```python
from build123d import *

# Parameters (mm, degrees)
F1_DEPTH = 2.54


with BuildPart() as f1:
    # F0 (on Top) → F1 (new body)
    with BuildSketch(Plane.XY):
        with BuildLine():
            ThreePointArc((-11.5484487595, -6.6675), (-11.5484487595, 6.6675), (0, 13.335))
            Line((0, 13.335), (0, 41.5238420934))
            ThreePointArc((0, 41.5238420934), (-3.4923003016, 43.8671250358), (-2.6478593482, 47.9870832663))
            ThreePointArc((-2.6478593482, 47.9870832663), (-4.0365508418, 49.1893730793), (-4.9196396151, 50.8))
            Line((-4.9196396151, 50.8), (-7.62, 50.8))
            ThreePointArc((-7.62, 50.8), (-13.2627477276, 7.6572509707), (-47.8040905122, -18.8008864232))
            Line((-47.8040905122, -18.8008864232), (-46.456170155, -21.1355529664))
            ThreePointArc((-46.456170155, -21.1355529664), (-44.598962502, -21.0983297604), (-42.8475396736, -21.7172998002))
            ThreePointArc((-42.8475396736, -21.7172998002), (-39.7349535137, -18.946869689), (-35.9932219183, -20.7806963635))
            Line((-35.9932219183, -20.7806963635), (-11.5484487595, -6.6675))
        make_face()
        with BuildLine():
            ThreePointArc((0, 13.335), (9.4292689271, 9.4292689271), (13.335, 0))
            ThreePointArc((13.335, 0), (12.8806208936, -3.4513519664), (11.5484487595, -6.6675))
            Line((11.5484487595, -6.6675), (35.1015943461, -20.2659149447))
            ThreePointArc((35.1015943461, -20.2659149447), (39.7899129003, -17.9160164205), (43.7992079136, -21.2965352321))
            ThreePointArc((43.7992079136, -21.2965352321), (45.116331258, -21.045134002), (46.4539103198, -21.1394671159))
            Line((46.4539103198, -21.1394671159), (47.8040905122, -18.8008864232))
            ThreePointArc((47.8040905122, -18.8008864232), (13.2627477276, 7.6572509707), (7.62, 50.8))
            Line((7.62, 50.8), (4.9241592856, 50.8))
            ThreePointArc((4.9241592856, 50.8), (4.0400398552, 49.1880973327), (2.6495579427, 47.9854097477))
            ThreePointArc((2.6495579427, 47.9854097477), (3.4815648437, 46.7545040826), (3.77400783, 45.2978499234))
            ThreePointArc((3.77400783, 45.2978499234), (2.6686265288, 42.6292233945), (0, 41.5238420934))
            Line((0, 41.5238420934), (0, 13.335))
        make_face()
        with BuildLine():
            ThreePointArc((-11.5484487595, -6.6675), (0, -13.335), (11.5484487595, -6.6675))
            Line((11.5484487595, -6.6675), (9.788685139, -5.6515))
            ThreePointArc((9.788685139, -5.6515), (0, -11.303), (-9.788685139, -5.6515))
            Line((-9.788685139, -5.6515), (-11.5484487595, -6.6675))
        make_face()
        with BuildLine():
            Line((35.1015943461, -20.2659149447), (11.5484487595, -6.6675))
            ThreePointArc((11.5484487595, -6.6675), (0, -13.335), (-11.5484487595, -6.6675))
            Line((-11.5484487595, -6.6675), (-35.9932219183, -20.7806963635))
            ThreePointArc((-35.9932219183, -20.7806963635), (-35.6199482657, -21.6818586781), (-35.4926315741, -22.6489249617))
            ThreePointArc((-35.4926315741, -22.6489249617), (-36.9699808664, -25.6250875678), (-40.2337772061, -26.2477738787))
            ThreePointArc((-40.2337772061, -26.2477738787), (-40.5740144012, -28.0722881249), (-41.5342707047, -29.6605328841))
            Line((-41.5342707047, -29.6605328841), (-40.1840905122, -31.9991135768))
            ThreePointArc((-40.1840905122, -31.9991135768), (0, -15.3145019414), (40.1840905122, -31.9991135768))
            Line((40.1840905122, -31.9991135768), (41.5320108695, -29.6644470336))
            ThreePointArc((41.5320108695, -29.6644470336), (40.7807919893, -28.5517697437), (40.3400163627, -27.2836619389))
            ThreePointArc((40.3400163627, -27.2836619389), (35.4097809691, -25.4998607522), (35.1015943461, -20.2659149447))
        make_face()
        with BuildLine():
            ThreePointArc((11.5484487595, -6.6675), (12.8806208936, -3.4513519664), (13.335, 0))
            ThreePointArc((13.335, 0), (9.4292689271, 9.4292689271), (0, 13.335))
            Line((0, 13.335), (0, 11.303))
            ThreePointArc((0, 11.303), (7.9924279478, 7.9924279478), (11.303, 0))
            ThreePointArc((11.303, 0), (10.9178596145, -2.9254316668), (9.788685139, -5.6515))
            Line((9.788685139, -5.6515), (11.5484487595, -6.6675))
        make_face()
        with BuildLine():
            Line((0, 11.303), (0, 13.335))
            ThreePointArc((0, 13.335), (-11.5484487595, 6.6675), (-11.5484487595, -6.6675))
            Line((-11.5484487595, -6.6675), (-9.788685139, -5.6515))
            ThreePointArc((-9.788685139, -5.6515), (-9.788685139, 5.6515), (0, 11.303))
        make_face()
    extrude(amount=F1_DEPTH)


solid = f1.part
```
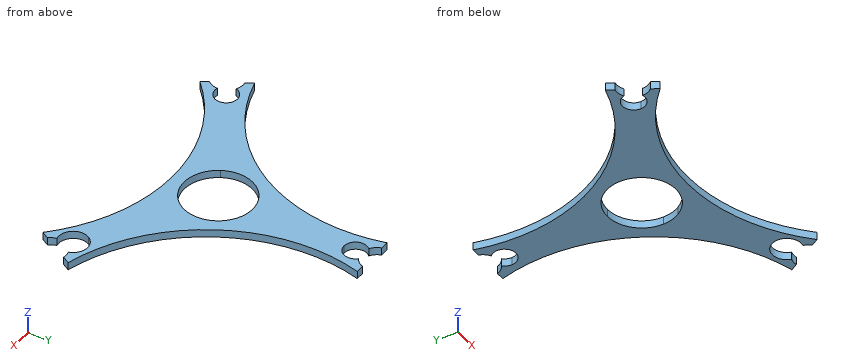
Can you work these out from the model? Positions are in its coordinate system, mm. Coordinates: 2 decimals unless noted, no trailing zeros. Order: outer loops, then holes, each group sorted by start corner. A loop starts at its lowest first (then second) coordinate and runs counter-clockwise, first axis right, second up.
1. If we section it at A-A (z = 2.05): Please give me the cut outline in (x, y) (1 decimal), then the cut area to 3 significant figures.
2. If we section it at C-C (x = 16.5): Please give me the cut outline in (y, z).
3. I need wall thicknesses on line 1 (X direction, y = -20, z = 2.45); line 2 (X direction, y = -6, z = 0.75); line 3 (X direction, y = -20.5, z = 0.4). Which ranges of each line are inside material? Lowest first, please.
4. I'm going to push flat-ended pins straight in: pin 1 (1.5 mm diameter, centred on x = 1.5, y = 32, fed in from -Z); pin 2 (1 mm diameter, centred on y = 12.5, z = 0.5, fed in from -X). Where does each tip first touch, or does it pass through?
5. If we section it at B-B (y = 34.5): Please give me the cut outline in (x, z).
Entries:
1. outline: (-47.8, -18.8) - (-46.5, -21.1) arc R5.2 cw to (-42.8, -21.7) arc R3.7 cw (long way) to (-40.2, -26.2) arc R5.2 cw to (-41.5, -29.7) - (-40.2, -32) arc R56.7 cw to (40.2, -32) - (41.5, -29.7) arc R5.2 cw to (40.3, -27.3) arc R4.8 cw (long way) to (43.8, -21.3) arc R5.2 cw to (46.5, -21.1) - (47.8, -18.8) arc R56.7 cw to (7.6, 50.8) - (4.9, 50.8) arc R5.2 cw to (2.6, 48) arc R3.8 cw (long way) to (-2.6, 48) arc R5.2 cw to (-4.9, 50.8) - (-7.6, 50.8) arc R56.7 cw to start; hole circle Ø22.6 at (0, 0)
1. area: 1,640 mm2
2. outline: (-17.77, 0) - (2.67, 0) - (2.67, 2.54) - (-17.77, 2.54) - close
3. line 1: x = -47.11 to -41.86, -36.59 to -22.58, 22.58 to 35.27, 43.19 to 47.11
3. line 2: x = -24.28 to -9.58, 9.58 to 24.28
3. line 3: x = -46.82 to -42.29, -36.17 to -23.7, 23.7 to 34.98, 43.48 to 46.82
4. pin 1: stops at z = 0
4. pin 2: stops at x = -11
5. outline: (-5.68, 0) - (5.68, 0) - (5.68, 2.54) - (-5.68, 2.54) - close
